```python
from build123d import *

# Parameters (mm, degrees)
SKETCH1_W                = 120
SKETCH1_H                = 70
SKETCH1_R                = 3
SKETCH1_W_2              = 12
SKETCH1_H_2              = 46
BOSS_EXTRUDE1_DEPTH      = 7.2
FILLET1_R                = 2
SKETCH2_W                = 120
SKETCH2_H                = 5
BOSS_EXTRUDE2_DEPTH      = 120
SKETCH9_W                = 7.2
SKETCH9_H                = 55
BOSS_EXTRUDE3_DEPTH      = 45
CUT_EXTRUDE5_DEPTH       = 167.442212194
CUT_EXTRUDE5_DEPTH_BACK  = 167.442212194
SKETCH10_R               = 5.5
SKETCH10_R_2             = 2
CUT_EXTRUDE4_DEPTH       = 4
CUT_EXTRUDE6_DEPTH       = 4
CUT_EXTRUDE7_DEPTH       = 4
SKETCH15_R               = 1.5
CUT_EXTRUDE8_DEPTH       = 7.2
CUT_EXTRUDE9_DEPTH       = 3.5
SKETCH17_W               = 7.2
SKETCH17_H               = 60
BOSS_EXTRUDE4_DEPTH      = 60
CUT_EXTRUDE10_DEPTH      = 141.249634581
CUT_EXTRUDE10_DEPTH_BACK = 141.249634581
SKETCH18_R               = 4
SKETCH19_R               = 1.5
CUT_EXTRUDE11_DEPTH      = 7.2
SKETCH20_R               = 8.5
CUT_EXTRUDE12_DEPTH      = 3
SKETCH21_R               = 19.175
CUT_EXTRUDE13_DEPTH      = 7.2


with BuildPart() as part:
    # Sketch1 → Boss-Extrude1 (new body)
    with BuildSketch(Plane(origin=(0, 0, 0), x_dir=(1, 0, 0), z_dir=(0, 1, 0))):
        Rectangle(SKETCH1_W, SKETCH1_H)
        with Locations(Location((-37.5, 24, 0), (0, 0, 270))):
            Circle(SKETCH1_R, mode=Mode.SUBTRACT)
        with Locations(Location((-37.5, -24, 0), (0, 0, 90))):
            Circle(SKETCH1_R, mode=Mode.SUBTRACT)
        with Locations(Location((37.5, 24, 0), (0, 0, 90))):
            Circle(SKETCH1_R, mode=Mode.SUBTRACT)
        with Locations(Location((37.5, -24, 0), (0, 0, 270))):
            Circle(SKETCH1_R, mode=Mode.SUBTRACT)
        Rectangle(SKETCH1_W_2, SKETCH1_H_2, mode=Mode.SUBTRACT)
    extrude(amount=BOSS_EXTRUDE1_DEPTH)

    # Fillet1
    fillet1_edges = [part.edges().sort_by_distance(p)[0] for p in [
        (-6, 3.6, -23),
        (-6, 3.6, 23),
        (6, 3.6, 23),
        (6, 3.6, -23),
    ]]
    fillet(fillet1_edges, radius=FILLET1_R)

    # Sketch2 → Boss-Extrude2 (add)
    with BuildSketch(Plane.XZ):
        with Locations((0, -32.5)):
            Rectangle(SKETCH2_W, SKETCH2_H)
    extrude(amount=BOSS_EXTRUDE2_DEPTH)

    # Sketch9 → Boss-Extrude3 (add)
    with BuildSketch(Plane.XY.offset(-30)):
        with Locations((-46.3, -27.5)):
            Rectangle(SKETCH9_W, SKETCH9_H)
        with Locations((46.3, -27.5)):
            Rectangle(SKETCH9_W, SKETCH9_H)
    extrude(amount=BOSS_EXTRUDE3_DEPTH)

    # Sketch10 → Cut-Extrude5 (cut, two sides: drawn at the far end of the back side and taken through both)
    with BuildSketch(Plane.ZY.offset(49.9).offset(-CUT_EXTRUDE5_DEPTH_BACK)):
        with Locations(Location((0, -27.5, 0), (0, 0, 270))):
            Circle(SKETCH10_R)
        with Locations(Location((0, -9, 0), (0, 0, 270))):
            Circle(SKETCH10_R_2)
        with Locations(Location((0, -46, 0), (0, 0, 270))):
            Circle(SKETCH10_R_2)
    extrude(amount=CUT_EXTRUDE5_DEPTH + CUT_EXTRUDE5_DEPTH_BACK, mode=Mode.SUBTRACT)

    # Sketch8 → Cut-Extrude4 (cut)
    with BuildSketch(Plane.XZ):
        Polygon((42.7, 27.0022214), (37.5, 30.0044428), (32.3, 27.0022214), (32.3, 20.9977786), (37.5, 17.9955572), (42.7, 20.9977786), align=None)
        Polygon((-32.3, 27.0022214), (-37.5, 30.0044428), (-42.7, 27.0022214), (-42.7, 20.9977786), (-37.5, 17.9955572), (-32.3, 20.9977786), align=None)
        Polygon((42.7, -20.9977786), (37.5, -17.9955572), (32.3, -20.9977786), (32.3, -27.0022214), (37.5, -30.0044428), (42.7, -27.0022214), align=None)
        Polygon((-32.3, -20.9977786), (-37.5, -17.9955572), (-42.7, -20.9977786), (-42.7, -27.0022214), (-37.5, -30.0044428), (-32.3, -27.0022214), align=None)
    extrude(amount=-CUT_EXTRUDE4_DEPTH, mode=Mode.SUBTRACT)

    # Sketch11 → Cut-Extrude6 (cut)
    with BuildSketch(Plane.ZY.offset(49.9)):
        Polygon((0, -13.849742261), (4.2, -11.424871131), (4.2, -6.575128869), (0, -4.150257739), (-4.2, -6.575128869), (-4.2, -11.424871131), align=None)
        Polygon((0, -50.849742261), (4.2, -48.424871131), (4.2, -43.575128869), (0, -41.150257739), (-4.2, -43.575128869), (-4.2, -48.424871131), align=None)
    extrude(amount=-CUT_EXTRUDE6_DEPTH, mode=Mode.SUBTRACT)

    # Sketch12 → Cut-Extrude7 (cut)
    with BuildSketch(Plane(origin=(49.9, 0, 0), x_dir=(0, 0, -1), z_dir=(1, 0, 0))):
        Polygon((0, -13.849742261), (4.2, -11.424871131), (4.2, -6.575128869), (0, -4.150257739), (-4.2, -6.575128869), (-4.2, -11.424871131), align=None)
        Polygon((0, -41.150257739), (-4.2, -43.575128869), (-4.2, -48.424871131), (0, -50.849742261), (4.2, -48.424871131), (4.2, -43.575128869), align=None)
    extrude(amount=-CUT_EXTRUDE7_DEPTH, mode=Mode.SUBTRACT)

    # Sketch15 → Cut-Extrude8 (cut)
    with BuildSketch(Plane.ZY.offset(49.9)):
        with Locations((0, -17.975)):
            Circle(SKETCH15_R)
        with Locations((0, -37.025)):
            Circle(SKETCH15_R)
    extrude(amount=-CUT_EXTRUDE8_DEPTH, mode=Mode.SUBTRACT)

    # Sketch16 → Cut-Extrude9 (cut)
    with BuildSketch(Plane(origin=(-42.7, 0, 0), x_dir=(0, 0, -1), z_dir=(1, 0, 0))):
        Polygon((1.732050808, -14.975), (-1.732050808, -14.975), (-3.464101615, -17.975), (-1.732050808, -20.975), (1.732050808, -20.975), (3.464101615, -17.975), align=None)
        Polygon((1.732050808, -34.025), (-1.732050808, -34.025), (-3.464101615, -37.025), (-1.732050808, -40.025), (1.732050808, -40.025), (3.464101615, -37.025), align=None)
    extrude(amount=-CUT_EXTRUDE9_DEPTH, mode=Mode.SUBTRACT)

    # Sketch17 → Boss-Extrude4 (add)
    with BuildSketch(Plane.XY.offset(-30)):
        with Locations((0, -85)):
            Rectangle(SKETCH17_W, SKETCH17_H)
        with Locations((-46.3, -85)):
            Rectangle(SKETCH17_W, SKETCH17_H)
    extrude(amount=BOSS_EXTRUDE4_DEPTH)

    # Sketch18 → Cut-Extrude10 (cut, two sides: drawn at the far end of the back side and taken through both)
    with BuildSketch(Plane(origin=(3.6, 0, 0), x_dir=(0, 0, -1), z_dir=(1, 0, 0)).offset(-CUT_EXTRUDE10_DEPTH_BACK)):
        with Locations(Location((0, -85, 0), (0, 0, 90))):
            Circle(SKETCH18_R)
    extrude(amount=CUT_EXTRUDE10_DEPTH + CUT_EXTRUDE10_DEPTH_BACK, mode=Mode.SUBTRACT)

    # Sketch19 → Cut-Extrude11 (cut)
    with BuildSketch(Plane(origin=(3.6, 0, 0), x_dir=(0, 0, -1), z_dir=(1, 0, 0))):
        with Locations(Location((0, -74, 0), (0, 0, 90))):
            Circle(SKETCH19_R)
        with Locations(Location((9.526279442, -79.5, 0), (0, 0, 90))):
            Circle(SKETCH19_R)
        with Locations(Location((9.526279442, -90.5, 0), (0, 0, 90))):
            Circle(SKETCH19_R)
        with Locations(Location((0, -96, 0), (0, 0, 90))):
            Circle(SKETCH19_R)
        with Locations(Location((-9.526279442, -90.5, 0), (0, 0, 90))):
            Circle(SKETCH19_R)
        with Locations(Location((-9.526279442, -79.5, 0), (0, 0, 90))):
            Circle(SKETCH19_R)
    extrude(amount=-CUT_EXTRUDE11_DEPTH, mode=Mode.SUBTRACT)

    # Sketch20 → Cut-Extrude12 (cut)
    with BuildSketch(Plane.ZY.offset(3.6)):
        with Locations(Location((0, -85, 0), (0, 0, 270))):
            Circle(SKETCH20_R)
    extrude(amount=-CUT_EXTRUDE12_DEPTH, mode=Mode.SUBTRACT)

    # Sketch21 → Cut-Extrude13 (cut)
    with BuildSketch(Plane.ZY.offset(49.9)):
        with Locations((0, -85)):
            Circle(SKETCH21_R)
    extrude(amount=-CUT_EXTRUDE13_DEPTH, mode=Mode.SUBTRACT)


solid = part.part
```
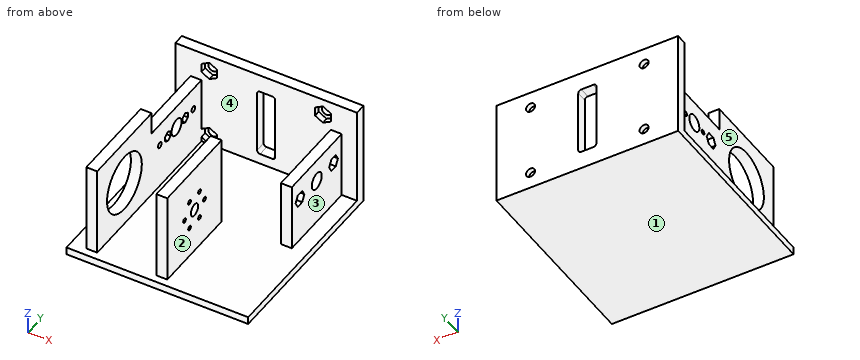
Geometry check sheet. Reference: the model listing, model coordinates, mm. Face numbers are marked on the shaded views. A direction names the side the tool comes from. Give positions to 0.01 mm unless a question says otherwise; leave off trailing zeros. Write each loop counter-clockwise with the first axis right and the second up, starting at its lowest first coordinate (ties: lowest second). Pieces come first, ordered by that corner, then holes. Notation, with made-up numbers: (-35, 59) - (10, 59) arc R21 ccw to (10, 67) - close; hole circle Ø1 at (-29, 69.5). An arc over 180 degrees is marked (long way). Use a Markdown table: item, result.
Q1. Set-up check for the marked faces 1 and 2: record each of +Z, -Z, +X, -X, +Y, -Y from which the full face is reachable in a straight line by a thin tool's end or side.
Computed:
| item | result |
|---|---|
| face 1 | -Z, +X, -X, +Y, -Y |
| face 2 | +Z, +X, -Y |
Q2. Thickness scan on L1, parallel to Y at x = 45, z = 0; L2, parallel to X at y = -96.5, z = 27.5; L3, parallel to X at y = -9.5, z = -3.5. Record the ranges inside material, lowest first. Write a range as [from, to].
Computed:
| item | result |
|---|---|
| L1 | y = [-55, -48], [-44, -33], [-22, -11], [-7, 7.2] |
| L2 | x = [-49.9, -42.7], [-3.6, 3.6] |
| L3 | x = [-45.9, -42.7], [42.7, 45.9] |
Q3. Draft check along X on the marked faces 3, 4 and 5. Enter one of: pulls with the +X half, pulls with the -X half, needs draft (parallel to the pull), parting line crosses it, or undercut.
Computed:
| item | result |
|---|---|
| face 3 | pulls with the +X half |
| face 4 | undercut |
| face 5 | pulls with the -X half |
Q4. Go/stop test with flat-tipped pins: P1, Ø13.5, axis at y = -18, z = -9, coming from the +X side; P2, Ø1.5, axis at x = 37.5, y = -97.5, coming from the +Z side; P3, Ø2, axis at x = 5.5, z = 25, coming from the -Y side. Record where each tip stops, or that it passes through.
Computed:
| item | result |
|---|---|
| P1 | stops at x = 49.9 |
| P2 | stops at z = -30 |
| P3 | stops at y = 0 |
Q5. Section check B-B, the plane x = -17. Enter the section's corners in (y, z), then the cut area to 3 significant figures.
Computed:
| item | result |
|---|---|
| outline | (-120, -35) - (7.2, -35) - (7.2, 35) - (0, 35) - (0, -30) - (-120, -30) - close |
| area | 1,100 mm² |
Q6. Section check A-A, the plane y = -85. Enter the section's corners in (x, z) (3 decimals), then the cut area to 3 significant figures.
Computed:
| item | result |
|---|---|
| outline | (-60, -35) - (60, -35) - (60, -30) - (3.6, -30) - (3.6, -4) - (-0.6, -4) - (-0.6, -8.5) - (-3.6, -8.5) - (-3.6, -30) - (-42.7, -30) - (-42.7, -19.175) - (-49.9, -19.175) - (-49.9, -30) - (-60, -30) - close; (-49.9, 19.175) - (-42.7, 19.175) - (-42.7, 30) - (-49.9, 30) - close; (-3.6, 8.5) - (-0.6, 8.5) - (-0.6, 4) - (3.6, 4) - (3.6, 30) - (-3.6, 30) - close |
| area | 1,100 mm² |
Q7. Section check C-C, the plane y = -57. Enter the section's corners in (x, z), then the cut area to 3 significant figures.
Computed:
| item | result |
|---|---|
| outline | (-60, -35) - (60, -35) - (60, -30) - (3.6, -30) - (3.6, 30) - (-3.6, 30) - (-3.6, -30) - (-42.7, -30) - (-42.7, 30) - (-49.9, 30) - (-49.9, -30) - (-60, -30) - close |
| area | 1,460 mm² |
